Geometry: final body of the model. Coordinates: model frame, mm. A direction names the side the tool comes from. Give positions to 0.01 mm unless a question says otherwise; leave off trailing zeros. Write each loop counter-clockwise with the first axis right and the second up, starting at its lowest first coordinate (ties: lowest second). Pieces come first, ordered by that corner, then holes. Notation, with made-up numbers: (-27, 52) -> (13, 52) arc R20 cw to (13, 75) -> close; hole circle Ø9 at (-33, 84). An arc over 180 degrees is marked (long way). Use CSV: the item, a comma, the result in double quotes. Start each with the question number.
1) Contact query for flat-ended pins moving along their axis: P1, Ø2.5, axis at x = 12, z = 2.5, coming from the +Y side; P2, Ø5, axis at y = -25, z = -61, coming from the -X side; P3, Ø6, axis at x = 8, z = -37.5, coming from the +Y side. Output: stop coordinate, or through.
2) Set-up query: faces 5 (the face through (50, -17, -113)), 6 (the face through (-38.498, 2.465, -125.408)). Return all of +Z, -Z, +X, -X, +Y, -Y with unobstructed straight access to the full face (end or side cutting, diameter ignored); none if empty.
3) Material intervals for line 1 (X direction, y = -0.5, z = -106); line 2 (Y direction, x = -12, z = -14); line 3 (X direction, y = -6, z = -37.5), sorted ascending. Write a range as [from, to].
4) Draft query along X for faces 1 (the face through (0.506, -22.986, -119.897)), 2 (the face through (-40, 5, -130)), 3 (the face through (34.32, -17.26, -38.83)), 4 (the face through (16.466, -2.958, 1.302)). Return one class per face: pulls with the +X half, pulls with the -X half, needs draft (parallel to the pull), parting line crosses it, or undercut.
5) Section A-A (x = -36.5). Output: boundary loops of the cut face in (y, z), plus the area to 3 significant figures.
6) Section B-B (y = -25.5). Output: boundary loops of the cut face in (x, z).
```python
from build123d import *

# Parameters (mm, degrees)
SKETCH2_W            = 150
SKETCH2_H            = 70
BOSS_EXTRUDE1_DEPTH  = 50
INTERSECT1_OUTLINE_W = 100
INTERSECT1_OUTLINE_H = 150
INTERSECT1_DEPTH     = 35
CUT_EXTRUDE1_DEPTH   = 153.887652053
SKETCH4_R            = 4
CUT_EXTRUDE3_DEPTH   = 6
SKETCH8_R            = 5
BOSS_EXTRUDE3_DEPTH  = 5


# Read off the part's stored shape, not the designer's step: Intersect1
with BuildPart() as part:
    # Sketch2 → Boss-Extrude1 (new, symmetric)
    with BuildSketch(Plane(origin=(0, 0, 0), x_dir=(0, 0, -1), z_dir=(1, 0, 0))):
        with Locations((65.177152604, 0)):
            Rectangle(SKETCH2_W, SKETCH2_H)
    extrude(amount=BOSS_EXTRUDE1_DEPTH, both=True)

    # Sketch1 → Cut-Revolve1 (revolve, cut)
    with BuildSketch(Plane(origin=(0, 0, 0), x_dir=(0, 0, -1), z_dir=(1, 0, 0)), mode=Mode.PRIVATE) as cut_revolve1_sk:
        with BuildLine():
            Line((140.177152604, 22.991315667), (100.177152604, 22.991315667))
            add(Edge.make_bspline(
                [(0, 0), (0.003001049, 0.012379499), (0.011197692, 0.036351162), (0.030910939, 0.072587893), (0.061826137, 0.121023529), (0.108056169, 0.183557631), (0.181890949, 0.271568579), (0.306591117, 0.401983994), (0.524430354, 0.601235581), (0.901337009, 0.902060291), (1.552737658, 1.35492318), (2.678502901, 2.03469009), (4.445764918, 2.96045388), (7.403328149, 4.31706154), (11.599431889, 5.985386832), (16.823063538, 7.814259146), (22.879973582, 9.705127394), (29.12300565, 11.472646372), (35.403551613, 13.101460315), (41.714266155, 14.60858848), (48.050573205, 16.004129586), (54.409190393, 17.293961353), (60.787889899, 18.480587367), (67.185029056, 19.563313869), (73.599488728, 20.538609835), (80.030497438, 21.398160754), (86.47762614, 22.128684831), (91.82278076, 22.603702016), (96.058091382, 22.875635683), (98.677996749, 22.971409991), (99.677383084, 22.991315667), (100.177152604, 22.991315667)],
                knots=[0, 0, 0, 0, 0, 0.000489987, 0.000979974, 0.001581787, 0.002219798, 0.003488078, 0.005411983, 0.008540376, 0.013605957, 0.022087023, 0.03601085, 0.059264391, 0.090564505, 0.147620712, 0.210220905, 0.272821133, 0.335421343, 0.398021557, 0.460621765, 0.523221981, 0.585822195, 0.648422407, 0.711022626, 0.773622837, 0.836223055, 0.89882327, 0.961423485, 0.980711742, 1, 1, 1, 1, 1], degree=4))
            Line((0, 0), (140.177152604, 0))
            Line((140.177152604, 0), (140.177152604, 22.991315667))
        make_face()
    revolve(cut_revolve1_sk.sketch.rotate(Axis((0, 0, 0), (0, 0, -1)), 90), axis=Axis((0, 0, 0), (0, 0, -1)), mode=Mode.SUBTRACT)

    # Intersect1 outline → Intersect1 (cut)
    with BuildSketch(Plane(origin=(0, 0, 0), x_dir=(1, 0, 0), z_dir=(0, 1, 0))):
        with Locations((0, 65.177152604)):
            Rectangle(INTERSECT1_OUTLINE_W, INTERSECT1_OUTLINE_H)
    extrude(amount=INTERSECT1_DEPTH, mode=Mode.SUBTRACT)

    # Sketch5 → Cut-Extrude1 (cut, through all)
    with BuildSketch(Plane(origin=(0, 0, 0), x_dir=(1, 0, 0), z_dir=(0, 1, 0))):
        Polygon((50, 86.137976919), (18.194421541, -9.822847396), (0, -21.198201401), (-18.194421541, -9.822847396), (-50, 86.137976919), (-75.365394844, 84.804131947), (-88.729692443, -46.913449713), (-13.099565549, -40.658440604), (76.90354762, -33.214709966), (74.65964276, 87.590776178), align=None)
    extrude(amount=-CUT_EXTRUDE1_DEPTH, mode=Mode.SUBTRACT)

    # Sketch4 → Cut-Extrude3 (cut)
    with BuildSketch(Plane(origin=(0, 0, 0), x_dir=(1, 0, 0), z_dir=(0, 1, 0))):
        with Locations(Location((12.5, -1.822847396, 0), (0, 0, 270))):
            Circle(SKETCH4_R)
    extrude(amount=-CUT_EXTRUDE3_DEPTH, mode=Mode.SUBTRACT)

    # Sketch8 → Boss-Extrude3 (add)
    with BuildSketch(Plane(origin=(0, 0, 0), x_dir=(1, 0, 0), z_dir=(0, 1, 0))):
        with Locations(Location((-40, 130.177152604, 0), (0, 0, 270))):
            Circle(SKETCH8_R)
    extrude(amount=BOSS_EXTRUDE3_DEPTH)


solid = part.part
```
Answers follow:
1,P1,"stops at y = -6"
1,P2,"stops at x = -42.5"
1,P3,"stops at y = -7.8"
2,face 5,"+Z, -Z, +X, +Y, -Y"
2,face 6,"+Y"
3,line 1,"x = [-50, -22.99], [22.99, 50]"
3,line 2,"y = [-35, 0]"
3,line 3,"x = [-33.88, -12.19], [12.19, 33.88]"
4,face 1,"undercut"
4,face 2,"needs draft"
4,face 3,"pulls with the +X half"
4,face 4,"undercut"
5,outline,"(-35, -140.18) -> (0, -140.18) -> (0, -133.75) -> (5, -133.75) -> (5, -126.61) -> (0, -126.61) -> (0, -45.41) -> (-35, -45.41) -> close"
5,area,"3,350 mm^2"
6,outline,"(-50, -140.18) -> (50, -140.18) -> (50, -86.14) -> (18.19, 9.82) -> (-18.19, 9.82) -> (-50, -86.14) -> close"
